Here's the drawing with two shaded views (mm, measured from the low corner). I have some questions. A direction names the side the tool comes from. Give positions to 0.01 mm unless a question says otherwise; leave off trailing zeros. Loops run counter-clockwise (first coordinate to the right, second up) from the corner with the lowest first, then second, coordinate; pieces in that order, holes last. Notation, with made-up numbers: (21, 8) -> (31, 8) arc R21 cw to (31, 45) -> close; hole circle Ø4 at (42.25, 29.25). An arc over 180 degrees is marked (long way). Answer in a Markdown table with one row per item. Add a question column.
Item 1: If we section it at A-A (y = 25.5): Write out the boundary of the cut face in (x, z).
Item 2: For P1, Ø20.5, axis at x = 68.5, y = 24, coming from the -Z side; P2, Ø4.5, axis at x = 80, z = 88.5, coming from the +Y side; P3, Ø6, axis at x = 59.5, z = 58, coming from the +Y side, each with a flat end and sliding along its axis, tell me the tip position at first contact or that it passes through.
Item 3: Which directions (+Z, -Z, +X, -X, +Y, -Y) give clear straight access to the entire face, cutting with the end or side of a thin tool? Please do the marked faces 1, 2 and 3.
Item 4: We'd pull the mould along Y, two halves only. Please class the marked faces 4, 5 and 6: released by +Y, released by -Y, zero draft, split by the parting line, or undercut.
Item 5: If we section it at B-B (x = 67): Write out the boundary of the cut face in (y, z), then the cut area to 3 significant figures.
Item 6: If we section it at C-C (x = 50.8): Write out the boundary of the cut face in (y, z), then the cut area to 3 significant figures.
Item 7: If I drill on line 1 (Z direction, x = 43.5, y = 18); line 2 (Z direction, x = 7, y = 51); line 3 (X direction, y = 32.5, z = 88) (1 decimal), over which ranges is the centre line in solid material (lowest first)?
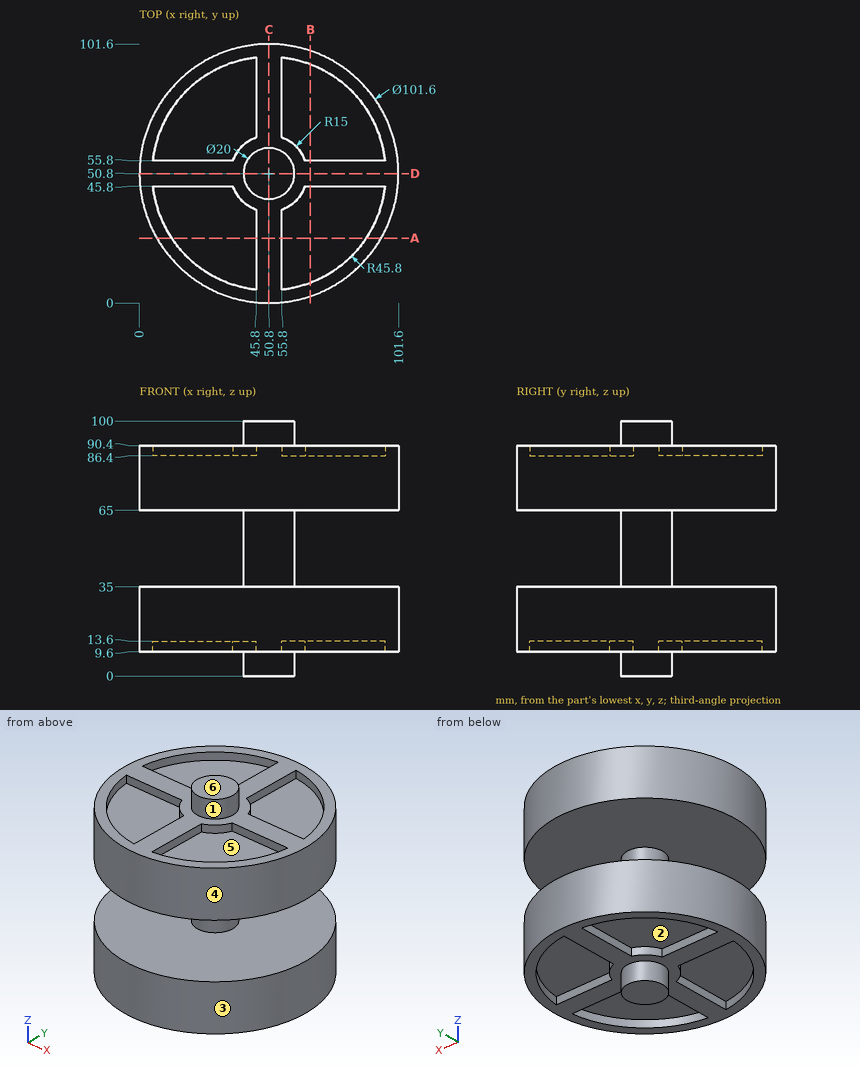
Recorded:
| question | item | result |
|---|---|---|
| 1 | outline | (6.75, 9.6) -> (12.62, 9.6) -> (12.62, 13.6) -> (45.8, 13.6) -> (45.8, 9.6) -> (55.8, 9.6) -> (55.8, 13.6) -> (88.98, 13.6) -> (88.98, 9.6) -> (94.85, 9.6) -> (94.85, 35) -> (6.75, 35) -> close; (6.75, 65) -> (94.85, 65) -> (94.85, 90.4) -> (88.98, 90.4) -> (88.98, 86.4) -> (55.8, 86.4) -> (55.8, 90.4) -> (45.8, 90.4) -> (45.8, 86.4) -> (12.62, 86.4) -> (12.62, 90.4) -> (6.75, 90.4) -> close |
| 2 | P1 | stops at z = 13.6 |
| 2 | P2 | stops at y = 93.86 |
| 2 | P3 | stops at y = 59.02 |
| 3 | face 1 | +Z |
| 3 | face 2 | -Z |
| 3 | face 3 | +Z, -Z |
| 4 | face 4 | split by the parting line |
| 4 | face 5 | undercut |
| 4 | face 6 | zero draft |
| 5 | outline | (2.65, 9.6) -> (7.96, 9.6) -> (7.96, 13.6) -> (45.8, 13.6) -> (45.8, 9.6) -> (55.8, 9.6) -> (55.8, 13.6) -> (93.64, 13.6) -> (93.64, 9.6) -> (98.95, 9.6) -> (98.95, 35) -> (2.65, 35) -> close; (2.65, 65) -> (98.95, 65) -> (98.95, 90.4) -> (93.64, 90.4) -> (93.64, 86.4) -> (55.8, 86.4) -> (55.8, 90.4) -> (45.8, 90.4) -> (45.8, 86.4) -> (7.96, 86.4) -> (7.96, 90.4) -> (2.65, 90.4) -> close |
| 5 | area | 4,290 mm^2 |
| 6 | outline | (0, 9.6) -> (40.8, 9.6) -> (40.8, 0) -> (60.8, 0) -> (60.8, 9.6) -> (101.6, 9.6) -> (101.6, 35) -> (60.8, 35) -> (60.8, 65) -> (101.6, 65) -> (101.6, 90.4) -> (60.8, 90.4) -> (60.8, 100) -> (40.8, 100) -> (40.8, 90.4) -> (0, 90.4) -> (0, 65) -> (40.8, 65) -> (40.8, 35) -> (0, 35) -> close |
| 6 | area | 6,150 mm^2 |
| 7 | line 1 | z = 13.6 to 35, 65 to 86.4 |
| 7 | line 2 | z = 9.6 to 35, 65 to 90.4 |
| 7 | line 3 | x = 3.4 to 8.8, 45.8 to 55.8, 92.8 to 98.2 |
